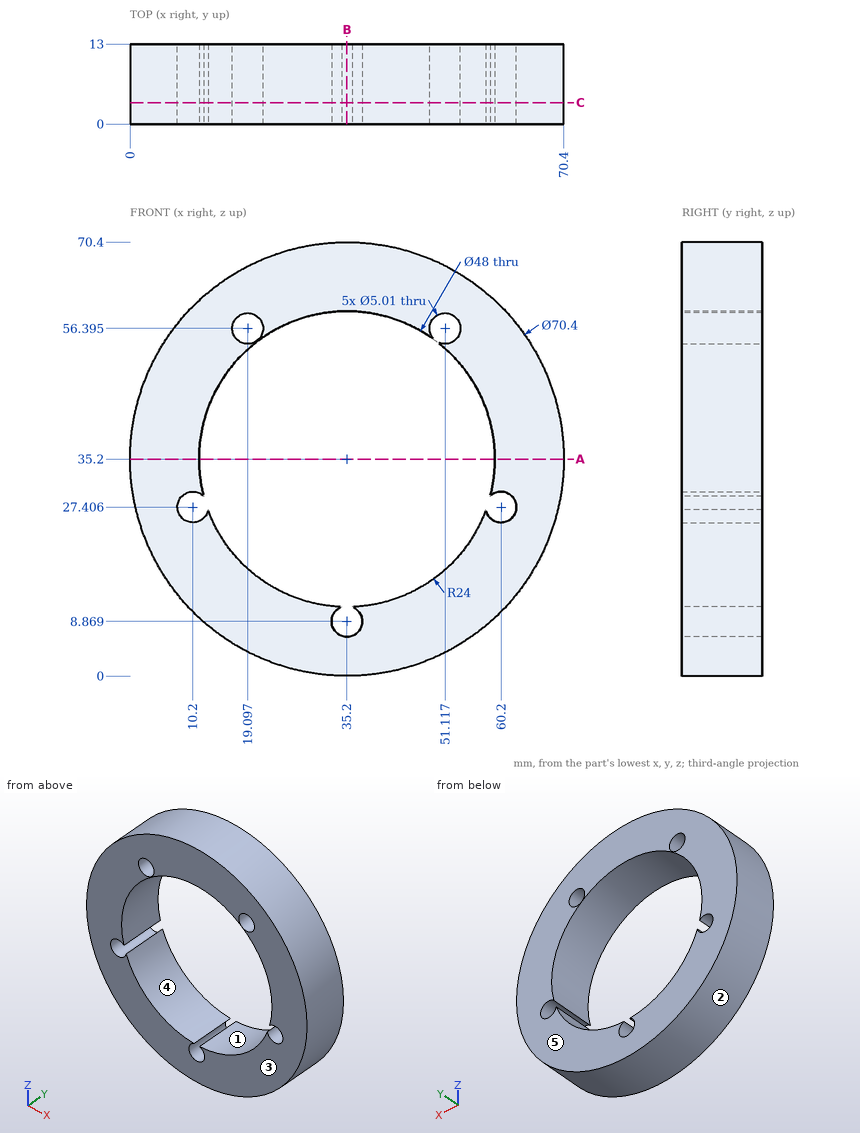
Input: dimensioned drawing with shaded views. Units: mm. Origin: part minimum x, y, z. A direction names the side the tool comes from. Give positions to 0.01 mm unless a question says otherwise; leave off trailing zeros. Loops run counter-clockwise (first coordinate to the right, second up) from the corner with the lowest first, then second, coordinate; pieces in that order, holes last. Notation, with made-up numbers: (26.25, 76.5) - (72.25, 76.5) arc R34 cw to (72.25, 115.5) - close; hole circle Ø7 at (48, 68). An arc over 180 degrees is marked (long way). Answer as CSV lines item,"result". Start each with the question number.
(1) Reachability of the marked faces 4 and 5 from +Z, -Z, +X, -X, +Y, -Y: full face, straight path, thin tool, end or side. Return the list, or none.
(2) Ray query, line 1 along X through (y, z) = (9.5, 29.5) (1 decimal); line 2 along X through (y, z) = (10.75, 35.2); line 3 along Z through (x, y) = (10.2, 10). Return the intervals inside material, ascending. Write a range as [from, to].
(3) Pin query (flat end, axial travel): P1, Ø4, axis at y = 9.5, z = 57, coming from the -X side; P2, Ø4, axis at x = 33.5, y = 3.5, coming from the +Z side; P3, Ø3, axis at y = 4, z = 48.5, coming from the +X side. Return the tip coordinate at first contact, or that it passes through.
(4) Mould query, pull axis X, two halves, no side actions, for the marked faces 1, 2 and 3. Classes: +X half, -X half, draft (parallel to the pull), parting line (faces both ways), or undercut.
(5) Section query A-A (z = 35.2). Output: boundary loops of the cut face in (x, y).
(6) Section query B-B (x = 35.2). Output: boundary loops of the cut face in (y, z) (1 decimal), and give its area (3 significant figures).
(7) Section query C-C (y = 3.5). Output: boundary loops of the cut face in (x, z) (1 decimal).
Worked answers:
1,face 4,"+Y, -Y"
1,face 5,"+Z, -Z, +X, -X, +Y"
2,line 1,"x = [0.5, 8.8], [11.6, 11.9], [58.5, 58.8], [61.6, 69.9]"
2,line 2,"x = [0, 11.2], [59.2, 70.4]"
2,line 3,"z = [10.42, 24.9], [29.91, 59.98]"
3,P1,"stops at x = 6.1"
3,P2,"stops at z = 70.4"
3,P3,"stops at x = 68.36"
4,face 1,"undercut"
4,face 2,"parting line"
4,face 3,"draft"
5,outline,"(0, 0) - (11.2, 0) - (11.2, 13) - (0, 13) - close; (59.2, 0) - (70.4, 0) - (70.4, 13) - (59.2, 13) - close"
6,outline,"(0, 0) - (13, 0) - (13, 6.4) - (0, 6.4) - close; (0, 59.2) - (13, 59.2) - (13, 70.4) - (0, 70.4) - close"
6,area,"228 mm^2"
7,outline,"circle Ø70.4 at (35.2, 35.2); hole (12, 29.2) arc R2.5 ccw (long way) to (12.7, 26.9) arc R24 ccw to (34.3, 11.2) arc R2.5 ccw (long way) to (36.1, 11.2) arc R24 ccw to (57.7, 26.9) arc R2.5 ccw (long way) to (58.4, 29.2) arc R24 ccw (long way) to start; hole circle Ø5 at (19.1, 56.4); hole circle Ø5 at (51.1, 56.4)"
